The model under review builds one solid part; all positions refer to its coordinate system, in mm. A direction names the side the tool comes from. Coordinates: 2 decimals unless noted, no trailing zeros. Write each loop counter-clockwise with the first axis right and the second up, starting at its lowest first coordinate (ties: lowest second). Pieces come first, ordered by that corner, then holes. Notation, with made-up numbers: (33, 31.5) - (81, 31.5) arc R20 cw to (81, 45.5) - close; hole circle Ø3 at (-30, 57). An arc over 180 degrees is marked (long way). Return JSON: item names as keys, results as strings. Group by question number.
(1) To check wall thickness, follow L1, parallel to Z at x = 0, y = -0.4; L2, parallel to Z at x = 60, y = -0.55; L3, parallel to X at y = 0.8, z = -1. State the ranges of each line that lie inside material, in increasing order. Write a range as from..to.
(2) We need section A-A on z = 0. State the section outline as (x, y) points.
(3) We need section B-B on y = -0.4. State the section outline as (x, z) points.
(4) Draft analysis for pull direction Z (two halves, no side actions). For faces 4 (the face through (10, 0, -6)), 5 (the face through (67, 0, 0)), 6 (the face through (55, 0, 0)), state which applies: released by +Z, released by -Z, zero draft, split by the parting line, or undercut.
(5) For pin 1 Ø0.9 at (x, y) = (5, -0.5) entering from +Z; pin 2 Ø1.8 at (x, z) = (0, 0) entering from -Y; pin 3 Ø1 at (y, z) = (0, -4) entering from -X, all flat-tipped, find the tip position at first contact; note any pin that passes through.
(6) Tool access review of faces 1 (the face through (-2.5, 0, -0.1)), 2 (the face through (10, 0, 6)), 3 (the face through (3, 0, -2.5)): name each direction out of +Z, -Z, +X, -X, +Y, -Y from which nothing blocks a thin tool from reaching the whole face with its end or side.
Solid Edge part; units mm, degrees
sketch "Sketch1" plane through (0, 0, 0) normal (0, -1, 0) x (1, 0, 0)
  circle A0 centre (0, 0) radius 1.5
  line L0 (0, 2.5) -> (10, 2.5)
  line L1 (10, 2.5) -> (10, 7)
  line L2 (10, 7) -> (60, 7)
  line L3 (10, -7) -> (60, -7)
  line L4 (10, -2.5) -> (10, -7)
  line L5 (0, -2.5) -> (10, -2.5)
  arc A1 (0, -2.5) -> (0, 2.5) centre (0, 0) cw
  arc A2 (60, 7) -> (60, -7) centre (60, 0) cw
  circle A3 centre (60, 0) radius 5
extrude "Protrusion1" add sketch "Sketch1" along normal mid plane 3
fillet "Redondeo_1" radius 3 2 edges at (10, 0, 2.5) (10, 0, -2.5)
properties part number "1976-1500-003" material "Aluminio, 7075-T6"
Ans:
{
 "1": {"L1": "-2.5..-1.5, 1.5..2.5", "L2": "-7..-5, 5..7", "L3": "-2.29..-1.12, 1.12..55.1, 64.9..66.93"},
 "2": {"outline": "(-2.5, -1.5) - (-1.5, -1.5) - (-1.5, 1.5) - (-2.5, 1.5) - close; (1.5, -1.5) - (55, -1.5) - (55, 1.5) - (1.5, 1.5) - close; (65, -1.5) - (67, -1.5) - (67, 1.5) - (65, 1.5) - close"},
 "3": {"outline": "(0, -2.5) - (7, -2.5) arc R3 cw to (10, -5.5) - (10, -7) - (60, -7) arc R7 ccw to (60, 7) - (10, 7) - (10, 5.5) arc R3 cw to (7, 2.5) - (0, 2.5) arc R2.5 ccw to start; hole circle Ø3 at (0, 0); hole circle Ø10 at (60, 0)"},
 "4": {"face 4": "zero draft", "face 5": "split by the parting line", "face 6": "undercut"},
 "5": {"pin 1": "z = 2.5", "pin 2": "through", "pin 3": "x = 9.24"},
 "6": {"face 1": "-X, +Y, -Y", "face 2": "+Z, -X, +Y, -Y", "face 3": "-Z, -X, +Y, -Y"}
}
